from build123d import *

# Parameters (mm, degrees)
REVOLVE1_ANGLE     = 360
SKETCH2_R          = 6.35
CUT_EXTRUDE1_DEPTH = 63.484
CIRPATTERN1_COUNT  = 5
CUT_EXTRUDE2_DEPTH = 7.62
CIRPATTERN2_COUNT  = 5


with BuildPart() as part:
    # Sketch1 → Revolve1 (revolve, symmetric)
    with BuildSketch(Plane.XY) as revolve1_sk:
        Polygon((32.512, 43.053), (38.1, 43.053), (38.1, 0), (80.645, 0), (80.645, -16.383), (31.75, -16.383), (31.75, -62.484), (25.4, -62.484), (25.4, -56.202878337), (20.567388856, -45.123813585), (22.706839799, -45.123813585), (22.706839799, -6.400010137), (26.858598141, 18.108781172), (25.922560718, 18.108781172), (30.977038212, 27.881202719), (30.977038212, 29.21), (32.512, 29.21), align=None)
    revolve(axis=Axis((0, 66.608222053, 0), (0, -1, 0)), revolution_arc=REVOLVE1_ANGLE / 2)
    revolve(revolve1_sk.sketch, axis=Axis((0, 66.608222053, 0), (0, 1, 0)), revolution_arc=REVOLVE1_ANGLE / 2)

    # Sketch2 → Cut-Extrude1 (cut, through all)
    with BuildSketch(Plane(origin=(0, 0, 0), x_dir=(1, 0, 0), z_dir=(0, 1, 0))):
        with Locations((0, -56.798909535)):
            Circle(SKETCH2_R)
    cut_extrude1 = extrude(amount=-CUT_EXTRUDE1_DEPTH, mode=Mode.SUBTRACT)

    # CirPattern1: Cut-Extrude1 ×5 about axis
    cirpattern1_axis = Axis((0, 0, 0), (0, 1, 0))
    for i in range(1, CIRPATTERN1_COUNT):
        add(cut_extrude1.rotate(cirpattern1_axis, i * 360 / CIRPATTERN1_COUNT), mode=Mode.SUBTRACT)

    # Sketch3 → Cut-Extrude2 (cut)
    with BuildSketch(Plane(origin=(0, 0, 0), x_dir=(1, 0, 0), z_dir=(0, 1, 0))):
        with BuildLine():
            Line((-25.816115671, 58.929202602), (-17.918089551, 47.780088903))
            ThreePointArc((-17.918089551, 47.780088903), (0, 38.514784655), (17.918089551, 47.780088903))
            Line((17.918089551, 47.780088903), (25.816115671, 58.929202602))
            ThreePointArc((25.816115671, 58.929202602), (26.666104709, 64.585415867), (22.622433381, 68.630654062))
            ThreePointArc((22.622433381, 68.630654062), (0, 72.263), (-22.622433381, 68.630654062))
            ThreePointArc((-22.622433381, 68.630654062), (-26.666104709, 64.585415867), (-25.816115671, 58.929202602))
        make_face()
    cut_extrude2 = extrude(amount=-CUT_EXTRUDE2_DEPTH, mode=Mode.SUBTRACT)

    # CirPattern2: Cut-Extrude2 ×5 about axis
    cirpattern2_axis = Axis((0, 0, 0), (0, 1, 0))
    for i in range(1, CIRPATTERN2_COUNT):
        add(cut_extrude2.rotate(cirpattern2_axis, i * 360 / CIRPATTERN2_COUNT), mode=Mode.SUBTRACT)


solid = part.part
Verification items for the finished model (mm, model axes). A direction names the side the tool comes from. Give positions to 0.01 mm unless a question says otherwise; leave off trailing zeros. Loops run counter-clockwise (first coordinate to the right, second up) from the corner with the lowest first, then second, coordinate; pieces in that order, holes last. Notation, with made-up numbers: (67.25, -12) - (108.25, -12) arc R12 cw to (108.25, 0) - close; hole circle Ø1 at (65.25, 25). An arc over 180 degrees is marked (long way). Write item = value, one per line. Start each with the question number.
Q1. Depth check by flat-ended pin: P1, Ø10, axis at x = -54.02, z = 17.55, coming from the -Y side (1 decimal); P2, Ø16.5, axis at x = 0, z = 56.8, coming from the +Y side; P3, Ø1.5, axis at y = -11.5, z = 32, coming from the -X side; P4, Ø6, axis at y = 5.5, z = 1.5, coming from the -X side. Enter the tip coordinate at first touch or a pass-through.
Q2. Mould release check, pull along Z, two halves, no side actions. Record for faces 1 (the face through (-53.1, -3.76, -45.32)), 2 (the face through (22.877, -3.757, 30.988)), 3 (the face through (-14.3, -62.484, -21.3)): released by +Z, released by -Z, zero draft, split by the parting line, or undercut.
Q3. Cross-section at B-B, the plane x = 0. State how many separate pieces and enclosed holes the cut face has, and give its area (4 significant figures).
Q4. Cross-section at C-C, the plane y = -34. Enter the section's corners in (x, z).
Q5. Tool access check on faces 4 (the face through (-48.96, -3.76, 30.28)), 5 (the face through (34.33, -8.08, -52.23)). Record the directions out of +Z, -Z, +X, -X, +Y, -Y that give a thin tool (end or side, any length) a straight path to the whole face; none if there is none.
Q6. Thickness scan on line 1 (X direction, y = -57, z = 0); line 2 (Z direction, x = 0, y = 32.75); line 3 (Z direction, x = -1, y = -33). Record the ranges inside material, lowest first.
Q7. Cross-section at A-A, the plane y = 35. Enter the section's corners in (x, z).
Answer key:
q1.P1 = through
q1.P2 = 0
q1.P3 = -74.34
q1.P4 = -38.1
q2.face_1 = undercut
q2.face_2 = undercut
q2.face_3 = zero draft
q3.separate_pieces = 3
q3.enclosed_holes = 0
q3.area = 3,045 mm^2
q4.outline = circle Ø63.5 at (0, 0); hole circle Ø45.41 at (0, 0)
q5.face_4 = +Y
q5.face_5 = +Y, -Y
q6.line_1 = -31.75 to -25.4, 25.4 to 31.75
q6.line_2 = -38.1 to -32.51, 32.51 to 38.1
q6.line_3 = -31.73 to -22.68, 22.68 to 31.73
q7.outline = circle Ø76.2 at (0, 0); hole circle Ø65.02 at (0, 0)
